Here's the drawing with two shaded views (mm, measured from the low corner). I have some questions. A direction names the side the tool comes from. Coordinates: 2 decimals unless noted, no trailing zeros. Loops run counter-clockwise (first coordinate to the right, second up) from the corner with the lowest first, then second, coordinate; pieces in that order, holes last. Notation, with made-up numbers: (-7, -27.5) - (12, -27.5) arc R27 ccw to (12, -1.5) - close; hole circle Ø7 at (-32.5, 87). An arc over 180 degrees is marked (long way). One line per item, written item: value. Start each with the question number.
(1) If we mould it in two halves opening along X, with no side actions, what happens to the marked faces 1, 2, 3 and 4? For each: pulls with the +X half, pulls with the -X half, needs draft (parallel to the pull), parting line crosses it, or undercut.
(2) If we section it at D-D on x = 8: Write out the boundary of the cut face in (y, z).
(3) If we section it at B-B on y = 13: Write out the boundary of the cut face in (x, z), then the cut area to 3 significant figures.
(4) If I drill on line 1 along X through (y, z) = (12.75, 4); line 2 along Z through (x, y) = (0.1, 5); line 3 along Y through (x, z) = (8.8, 5), over which ranges is the centre line in solid material (lowest first)? Write a range as from..to.
(5) I'm going to push flat-ended pins straight in: P1, Ø2, axis at x = 2.5, y = 6.5, coming from the -Z side; P2, Ø1.5, axis at x = 1.5, z = 2.5, coming from the -Y side. Where does each tip first touch, or does it pass through?
(6) If we section it at C-C on y = 7.5: Write out the boundary of the cut face in (x, z).
(7) On a 3-axis mill with a long thin cutter (end or side, diameter ignored), from which of +Z, -Z, +X, -X, +Y, -Y can I reach the whole of each face in a straight line? I mean the marked faces 5 and 6. Say none if no direction works.
(8) If we section it at A-A on z = 5: Write out the boundary of the cut face in (x, y), then the cut area to 3 significant figures.
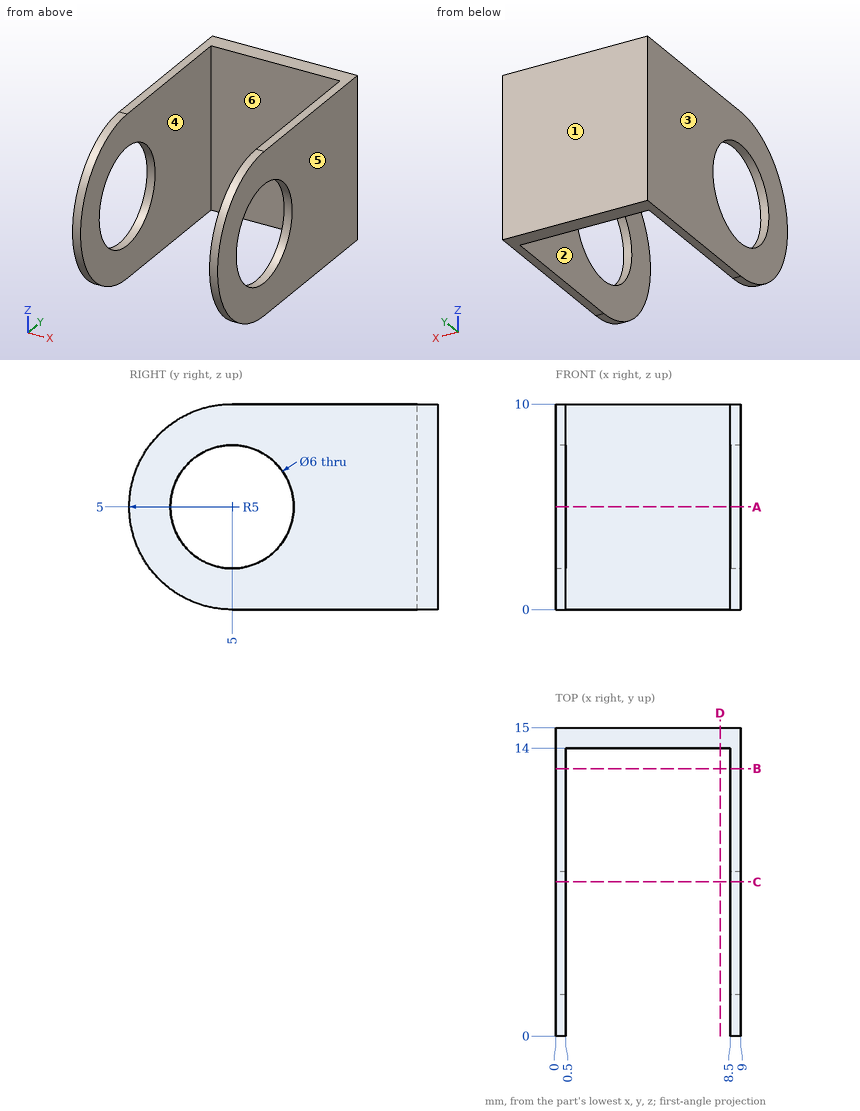
Values:
1. face 1: needs draft
1. face 2: undercut
1. face 3: pulls with the -X half
1. face 4: undercut
2. outline: (14, 0) - (15, 0) - (15, 10) - (14, 10) - close
3. outline: (0, 0) - (0.5, 0) - (0.5, 10) - (0, 10) - close; (8.5, 0) - (9, 0) - (9, 10) - (8.5, 10) - close
3. area: 10.0 mm2
4. line 1: x = 0..0.5, 8.5..9
4. line 2: z = 0..2, 8..10
4. line 3: y = 0..2, 8..15
5. P1: passes through
5. P2: stops at y = 14
6. outline: (0, 0) - (0.5, 0) - (0.5, 3.34) - (0, 3.34) - close; (0, 6.66) - (0.5, 6.66) - (0.5, 10) - (0, 10) - close; (8.5, 0) - (9, 0) - (9, 3.34) - (8.5, 3.34) - close; (8.5, 6.66) - (9, 6.66) - (9, 10) - (8.5, 10) - close
7. face 5: +Z, -Z, +X, +Y, -Y
7. face 6: +Z, -Z, -Y
8. outline: (0, 0) - (0.5, 0) - (0.5, 2) - (0, 2) - close; (0, 8) - (0.5, 8) - (0.5, 14) - (8.5, 14) - (8.5, 8) - (9, 8) - (9, 15) - (0, 15) - close; (8.5, 0) - (9, 0) - (9, 2) - (8.5, 2) - close
8. area: 17.0 mm2
